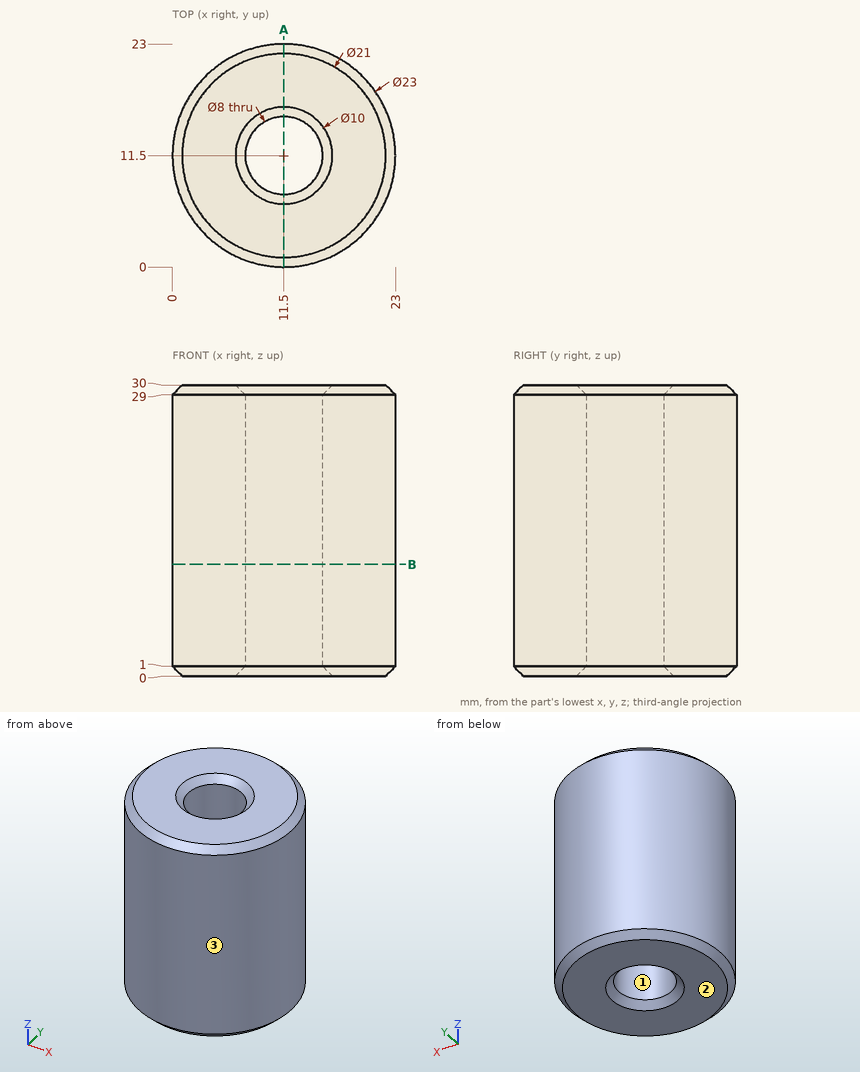
Design review of the part shown in the three views and the two pictorial views. Dimensions are in mm from the part's minimum x, y and z. Round coordinates to 2 decimals unless told otherwise and drop trailing zeros. Order: outer loops, then holes, each group sorted by start corner. A loop starts at its lowest first (then second) coordinate and runs counter-clockwise, first axis right, second up. Notation, with made-up numbers: (-28, 87.25) - (13, 87.25) arc R18 cw to (13, 92.25) - close; hole circle Ø1 at (23.25, -11). An arc over 180 degrees is marked (long way). One line per question, with ' | ' between items.
Item 1: Wall thickness on line 1 (Y direction, x = 11.5, z = 10); line 2 (X direction, y = 8.5, z = 15.5); line 3 (Y direction, x = 14, z = 13.25): over which ranges is each line inside the solid? List them lowest first. Write a range as [from, to].
Checks:
line 1: [0, 7.5], [15.5, 23] | line 2: [0.4, 8.85], [14.15, 22.6] | line 3: [0.28, 8.38], [14.62, 22.72]
Item 2: For P1, Ø1, axis at x = 7, z = 22, coming from the +Y side; P2, Ø5, axis at x = 14.5, y = 3.5, coming from the -Z side; P3, Ø1.5, axis at x = 9, z = 4, coming from the +Y side; P4, Ø8, axis at y = 6, z = 8, coming from the +X side, all flat-tipped, find the tip position at first contact; note any pin that passes through.
Checks:
P1: y = 22.28 | P2: z = 0 | P3: y = 22.87 | P4: x = 22.9
Item 3: Draft analysis for pull direction Y (two halves, no side actions). For the marked faces 1, 2 and 3, state which applies: +Y half, -Y half, draft (parallel to the pull), parting line (faces both ways), or undercut.
Checks:
face 1: undercut | face 2: draft | face 3: parting line
Item 4: Take a section at B-B, the plane z = 11.5. Write out the cut boundary in (x, y).
Checks:
outline: circle Ø23 at (11.5, 11.5); hole circle Ø8 at (11.5, 11.5)
Item 5: Take a section at A-A, the plane x = 11.5. Write out the cut boundary in (y, z).
Checks:
outline: (0, 1) - (1, 0) - (6.5, 0) - (7.5, 1) - (7.5, 29) - (6.5, 30) - (1, 30) - (0, 29) - close; (15.5, 1) - (16.5, 0) - (22, 0) - (23, 1) - (23, 29) - (22, 30) - (16.5, 30) - (15.5, 29) - close
